The model under review builds one solid part; all positions refer to its coordinate system, in mm. A direction names the side the tool comes from. Give positions to 0.01 mm unless a question says otherwise; leave off trailing zeros. Loops run counter-clockwise (first coordinate to the right, second up) from the corner with the lowest first, then second, coordinate; pieces in that order, holes last. Notation, with made-up numbers: (-0.5, 27) - (24.5, 27) arc R18 cw to (24.5, 45) - close; hole circle Ø5 at (-6, 55). An arc over 180 degrees is marked (long way). Return JSON: item names as keys, results as strings. Group by question number.
from build123d import *

# Parameters (mm, degrees)
CROQUIS1_W              = 295
CROQUIS1_H              = 152.4
SALIENTE_EXTRUIR1_DEPTH = 3.175
CROQUIS2_R              = 9
CROQUIS2_R_2            = 22.5
CROQUIS2_R_3            = 2
CROQUIS2_R_4            = 1.25
CORTAR_EXTRUIR1_DEPTH   = 3.175
CROQUIS3_R              = 1.25
CORTAR_EXTRUIR2_DEPTH   = 167.050506247


with BuildPart() as part:
    # Croquis1 → Saliente-Extruir1 (new body)
    with BuildSketch(Plane(origin=(0, 0, 0), x_dir=(1, 0, 0), z_dir=(0, 1, 0))):
        Rectangle(CROQUIS1_W, CROQUIS1_H)
    extrude(amount=SALIENTE_EXTRUIR1_DEPTH)

    # Croquis2 → Cortar-Extruir1 (cut)
    with BuildSketch(Plane(origin=(0, 3.175, 0), x_dir=(1, 0, 0), z_dir=(0, 1, 0))):
        with BuildLine():
            Line((-137.3, 55.8), (-137.3, 45.8))
            ThreePointArc((-137.3, 45.8), (-134.8, 43.3), (-132.3, 45.8))
            Line((-132.3, 45.8), (-132.3, 55.8))
            ThreePointArc((-132.3, 55.8), (-134.8, 58.3), (-137.3, 55.8))
        make_face()
        with BuildLine():
            ThreePointArc((-137.3, -45.8), (-134.8, -43.3), (-132.3, -45.8))
            Line((-132.3, -45.8), (-132.3, -55.8))
            ThreePointArc((-132.3, -55.8), (-134.8, -58.3), (-137.3, -55.8))
            Line((-137.3, -55.8), (-137.3, -45.8))
        make_face()
        with Locations((0, -31.8)):
            Circle(CROQUIS2_R)
        with Locations((96.12881982, 23.7)):
            Circle(CROQUIS2_R_2)
        with Locations(Location((53.548724126, 39.530889132, 0), (0, 0, 270))):
            Circle(CROQUIS2_R_3)
        with Locations(Location((88.548724126, -21.090889132, 0), (0, 0, 270))):
            Circle(CROQUIS2_R_3)
        with BuildLine():
            ThreePointArc((137.3, 45.8), (134.8, 43.3), (132.3, 45.8))
            Line((132.3, 45.8), (132.3, 55.8))
            ThreePointArc((132.3, 55.8), (134.8, 58.3), (137.3, 55.8))
            Line((137.3, 55.8), (137.3, 45.8))
        make_face()
        with BuildLine():
            Line((137.3, -55.8), (137.3, -45.8))
            ThreePointArc((137.3, -45.8), (134.8, -43.3), (132.3, -45.8))
            Line((132.3, -45.8), (132.3, -55.8))
            ThreePointArc((132.3, -55.8), (134.8, -58.3), (137.3, -55.8))
        make_face()
        with BuildLine():
            Line((82.592466968, 41.672677916), (-5.414541141, -24.610928834))
            ThreePointArc((-5.414541141, -24.610928834), (4.01678539, -23.746091934), (9, -31.8))
            ThreePointArc((9, -31.8), (7.505592222, -36.76649629), (3.518647689, -40.083665761))
            Line((3.518647689, -40.083665761), (104.925439043, 2.990835598))
            ThreePointArc((104.925439043, 2.990835598), (76.643248235, 12.45), (82.592466968, 41.672677916))
        make_face()
        with Locations(Location((-45.249827348, -57.925, 0), (0, 0, 270))):
            Circle(CROQUIS2_R_4)
    extrude(amount=-CORTAR_EXTRUIR1_DEPTH, mode=Mode.SUBTRACT)

    # Croquis3 → Cortar-Extruir2 (cut, through all)
    with BuildSketch(Plane(origin=(0, 3.175, 0), x_dir=(1, 0, 0), z_dir=(0, 1, 0))):
        with Locations(Location((0, -16.8, 0), (0, 0, 270))):
            Circle(CROQUIS3_R)
        with Locations(Location((12.990381057, -39.3, 0), (0, 0, 270))):
            Circle(CROQUIS3_R)
        with Locations(Location((-12.990381057, -39.3, 0), (0, 0, 270))):
            Circle(CROQUIS3_R)
        with BuildLine():
            Line((-52.334936491, 2.051152423), (-46.334936491, -8.341152423))
            ThreePointArc((-46.334936491, -8.341152423), (-47.25, -11.756215932), (-50.665063509, -10.841152423))
            Line((-50.665063509, -10.841152423), (-56.665063509, -0.448847577))
            ThreePointArc((-56.665063509, -0.448847577), (-55.75, 2.966215932), (-52.334936491, 2.051152423))
        make_face()
        with BuildLine():
            Line((-71, -15.3), (-68.5, -15.3))
            ThreePointArc((-68.5, -15.3), (-67, -16.8), (-68.5, -18.3))
            Line((-68.5, -18.3), (-71, -18.3))
            ThreePointArc((-71, -18.3), (-72.5, -16.8), (-71, -15.3))
        make_face()
        with BuildLine():
            Line((-58.009618943, -37.8), (-55.509618943, -37.8))
            ThreePointArc((-55.509618943, -37.8), (-54.009618943, -39.3), (-55.509618943, -40.8))
            Line((-55.509618943, -40.8), (-58.009618943, -40.8))
            ThreePointArc((-58.009618943, -40.8), (-59.509618943, -39.3), (-58.009618943, -37.8))
        make_face()
        with BuildLine():
            Line((-83.990381057, -37.8), (-81.490381057, -37.8))
            ThreePointArc((-81.490381057, -37.8), (-79.990381057, -39.3), (-81.490381057, -40.8))
            Line((-81.490381057, -40.8), (-83.990381057, -40.8))
            ThreePointArc((-83.990381057, -40.8), (-85.490381057, -39.3), (-83.990381057, -37.8))
        make_face()
        with BuildLine():
            Line((-71, -21.75), (-68.5, -21.75))
            ThreePointArc((-68.5, -21.75), (-58.45, -31.8), (-68.5, -41.85))
            Line((-68.5, -41.85), (-71, -41.85))
            ThreePointArc((-71, -41.85), (-81.05, -31.8), (-71, -21.75))
        make_face()
    extrude(amount=-CORTAR_EXTRUIR2_DEPTH, mode=Mode.SUBTRACT)


solid = part.part
Item 1: Take a section at B-B (y = 2.3). State how many separate pieces and enclosed holes the cut face has, then the cut area to 3 significant figures.
Item 2: Tool access review of faces 1 (the face through (-49.38, 1.61, 3.07)), 2 (the face through (-2, 0, -1)): name each direction out of +Z, -Z, +X, -X, +Y, -Y from which nothing blocks a thin tool from reaching the whole face with its end or side.
Item 3: Take a section at A-A (z = -23.7). State the section outline as (x, y) points (3 decimals).
Item 4: Mouldability with a two-part tool opening along Z and no side actions: class faces 3 (the face through (-2, 3.175, -1)), 4 (the face through (-7.884, 1.61, 36.141)), 5 (the face through (39.205, 1.61, -8.995)) as +Z half, -Z half, draft (parallel to the pull), parting line (faces both ways), or undercut.
Item 5: For L1, parallel to X at y = 2.8, z = 57; L2, parallel to X at y = 0.2, z = 29; L3, parallel to X at y = 2.5, z = 4.5, list the stretches that pass through material, from the lowest coordinate up. Write a range as from..to.
Check sheet entries:
{
 "1": {"separate pieces": "1", "enclosed holes": "16", "area": "39,700 mm^2"},
 "2": {"face 1": "+Y, -Y", "face 2": "+Z, -Z, +X, -X, -Y"},
 "3": {"outline": "(-147.5, 0) - (58.73, 0) - (58.73, 3.175) - (-147.5, 3.175) - close; (118.629, 0) - (147.5, 0) - (147.5, 3.175) - (118.629, 3.175) - close"},
 "4": {"face 3": "draft", "face 4": "undercut", "face 5": "undercut"},
 "5": {"L1": "x = -147.5..-136.99, -132.61..-46.09, -44.41..132.61, 136.99..147.5", "L2": "x = -147.5..-80.65, -58.85..-8.55, 29.61..147.5", "L3": "x = -147.5..-54.33, -48.55..21.29, 87.29..147.5"}
}
